Input: part model. Units: mm. Frame: model coordinates. A direction names the side the tool comes from. Coordinates: 2 decimals unless noted, no trailing zeros. Order: outer loops, then holes, each group sorted by start corner. A loop starts at its lowest first (then second) coordinate and runs counter-clockwise, first axis right, second up. Notation, with made-up numbers: (13.25, -6) -> (37.25, -6) arc R10 ccw to (37.25, -2) -> close; hole circle Ø11 at (-25, 53.5). An arc over 180 degrees is marked (long way). Write each question's results on one line, items separated by ' | '.
Autodesk Inventor part; units mm, degrees
ref_plane "YZ Plane" through (0, 0, 0) normal (1, 0, 0) x (0, 1, 0)
ref_plane "XZ Plane" through (0, 0, 0) normal (0, 1, 0) x (-1, 0, 0)
ref_plane "XY Plane" through (0, 0, 0) normal (0, 0, 1) x (1, 0, 0)
sketch "스케치1" plane through (0, 0, 0) normal (0, 0, 1) x (1, 0, 0)
  line L0 (-3, 0) -> (-1.5, 2.5981)
  line L1 (-1.5, 2.5981) -> (1.5, 2.5981)
  line L2 (1.5, 2.5981) -> (3, 0)
  line L3 (3, 0) -> (1.5, -2.5981)
  line L4 (1.5, -2.5981) -> (-1.5, -2.5981)
  line L5 (-1.5, -2.5981) -> (-3, 0)
  point P0 (0, 0)
  point P1 (0, 0)
  dimension "d0" = 6
extrude "돌출1" add sketch "스케치1" along normal blind 50
sketch "스케치2" plane through (0, 0, 50) normal (0, 0, 1) x (1, 0, 0)
  circle A0 centre (0, 0) radius 1.5
  dimension "d3" = 3
extrude "돌출2" add sketch "스케치2" along normal blind 5
sketch "스케치3" plane through (0, 0, 0) normal (0, 0, -1) x (-1, 0, 0)
  circle A0 centre (0, 0) radius 1.5
  dimension "d6" = 3
extrude "돌출3" cut sketch "스케치3" against normal blind 5
properties part number "50mm지지대"
(1) Pin query (flat end, axial travel): P1, Ø3, axis at y = 1, z = 26.5, coming from the -X side. Return the tip coordinate at first contact, or that it passes through.
Return value:
P1: x = -3
(2) Cut plane A-A, the plane x = 0. Return loops of the section in (y, z), plus the area to 3 significant figures.
Return value:
outline: (-2.6, 0) -> (-1.5, 0) -> (-1.5, 5) -> (1.5, 5) -> (1.5, 0) -> (2.6, 0) -> (2.6, 50) -> (1.5, 50) -> (1.5, 55) -> (-1.5, 55) -> (-1.5, 50) -> (-2.6, 50) -> close | area: 260 mm2
(3) Cut plane B-B, the plane z = 25.5. Return loops of the section in (x, y), plus the area to 3 significant figures.
Return value:
outline: (-3, 0) -> (-1.5, -2.6) -> (1.5, -2.6) -> (3, 0) -> (1.5, 2.6) -> (-1.5, 2.6) -> close | area: 23.4 mm2
(4) Cut plane C-C, the plane x = -2.4. Return loops of the section in (y, z), plus the area to 3 significant figures.
Return value:
outline: (-1.04, 0) -> (1.04, 0) -> (1.04, 50) -> (-1.04, 50) -> close | area: 104 mm2
(5) Reachability of faces 5 (the face through (1.5, 0.07, 2.46)), 6 (the face through (1.3, 1.2, 50)), 7 (the face through (0, 0, 55)) from +Z, -Z, +X, -X, +Y, -Y: full face, straight path, thin tool, end or side. Return the list, or none.
Return value:
face 5: -Z | face 6: +Z | face 7: +Z, +X, -X, +Y, -Y
(6) Line query: line 1 along Y through (x, z) = (0, 1.4); line 2 along Z through (x, y) = (-1.35, -1.4); line 3 along X through (y, z) = (1.4, 26.5). Output: solid intervals per line, ascending. Write a range as from..to.
Return value:
line 1: -2.6..-1.5, 1.5..2.6 | line 2: 0..50 | line 3: -2.19..2.19
(7) Mould query, pull axis Y, two halves, no side actions, for faces 1 (the face through (2.24, 1.32, 24.65)), 2 (the face through (0, 0, 5)), 3 (the face through (2.26, -1.28, 24.65)), 4 (the face through (-1.5, -0.07, 52.46)). Classes: +Y half, -Y half, draft (parallel to the pull), parting line (faces both ways), or undercut.
Return value:
face 1: +Y half | face 2: undercut | face 3: -Y half | face 4: parting line
